Could you check a few things on this model? Use its own coordinates, in mm. Face numbers are marked on the shaded views. A direction names the side the tool comes from. Coordinates: 2 decimals unless noted, no trailing zeros. Order: outer loops, then holes, each group sorted by start corner. A loop starts at its lowest first (then second) coordinate and runs counter-clockwise, first axis right, second up. Notation, with made-up numbers: (-18.75, 80) - (-7.75, 80) arc R30 cw to (-7.75, 113) - close; hole circle Ø10 at (50.5, -30.5). An arc over 180 degrees is marked (long way). Answer as a JSON object with one key per item and string values. Group by question number.
(1) Imagine slicing it at C-C, the plane y = 118. Write out the boundary of the cut face in (x, z), and give its area (3 significant figures).
(2) Please list where these lines run through material, in increasing order: probe 1 along Y at (x, z) = (-6.5, 11); probe 2 along X at (y, z) = (48, -6); probe 3 along X at (y, z) = (30.5, 10).
(3) Imagine slicing it at D-D, the plane x = 8. Write out the boundary of the cut face in (y, z), and give its area (3 significant figures).
(4) Which directions (+Z, -Z, +X, -X, +Y, -Y) give clear straight access to the entire face, cutting with the end or side of a thin tool? Please do the marked faces 1 and 2.
(5) Imagine slicing it at A-A, the plane z = 0. Write out the boundary of the cut face in (x, y), and give its area (3 significant figures).
(6) Will these pins go through, and if not, where does the flat tip stop? P1, Ø17.5, axis at y = 44.5, z = 1, coming from the -X side; P2, Ø6, axis at x = 11, y = 96.5, coming from the +Z side; P3, Ø11, axis at y = 41, z = 1.5, coming from the +X side.
(7) Imagine slicing it at B-B, the plane x = 1.5. Write out the boundary of the cut face in (y, z), and give its area (3 significant figures).
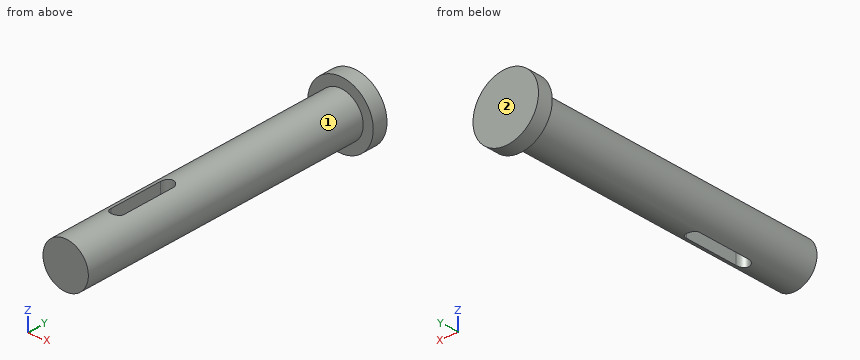
from build123d import *

# Parameters (mm, degrees)
SKETCH1_R           = 11.43
BOSS_EXTRUDE1_DEPTH = 160.02
CUT_EXTRUDE1_DEPTH  = 73.66
BOSS_EXTRUDE2_START = -7.62
SKETCH3_R           = 16.51
SKETCH3_R_2         = 11.43
BOSS_EXTRUDE2_DEPTH = 7.62


with BuildPart() as part:
    # Sketch1 → Boss-Extrude1 (new body)
    with BuildSketch(Plane(origin=(0, 0, 0), x_dir=(1, 0, 0), z_dir=(0, 1, 0))):
        with Locations(Location((0, 0, 0), (0, 0, 270))):
            Circle(SKETCH1_R)
    extrude(amount=BOSS_EXTRUDE1_DEPTH)

    # Sketch2 → Cut-Extrude1 (cut)
    with BuildSketch(Plane.XY.offset(11.43)):
        with BuildLine():
            Line((3.301999683, 28.702000653), (3.301999683, 56.13399967))
            ThreePointArc((3.301999683, 56.13399967), (0, 59.436), (-3.302000317, 56.134000304))
            Line((-3.302000317, 56.134000304), (-3.302000317, 28.702000019))
            ThreePointArc((-3.302000317, 28.702000019), (0, 25.4), (3.301999683, 28.702000653))
        make_face()
    extrude(amount=-CUT_EXTRUDE1_DEPTH, mode=Mode.SUBTRACT)

    # Sketch3 → Boss-Extrude2 (add)
    with BuildSketch(Plane(origin=(0, 160.02, 0), x_dir=(1, 0, 0), z_dir=(0, 1, 0)).offset(BOSS_EXTRUDE2_START)):
        with Locations(Location((0, 0, 0), (0, 0, 270))):
            Circle(SKETCH3_R)
        with Locations(Location((0, 0, 0), (0, 0, 270))):
            Circle(SKETCH3_R_2, mode=Mode.SUBTRACT)
    extrude(amount=BOSS_EXTRUDE2_DEPTH)


solid = part.part
Result set:
{
 "1": {"outline": "circle Ø22.86 at (0, 0)", "area": "410 mm^2"},
 "2": {"probe 1": "y = 152.4 to 160.02", "probe 2": "x = -9.73 to -3.3, 3.3 to 9.73", "probe 3": "x = -5.54 to -3.3, 3.3 to 5.54"},
 "3": {"outline": "(0, -8.16) - (152.4, -8.16) - (152.4, -14.44) - (160.02, -14.44) - (160.02, 14.44) - (152.4, 14.44) - (152.4, 8.16) - (0, 8.16) - close", "area": "2,710 mm^2"},
 "4": {"face 1": "-Y", "face 2": "+Z, -Z, +X, -X, +Y"},
 "5": {"outline": "(-16.51, 152.4) - (-11.43, 152.4) - (-11.43, 0) - (11.43, 0) - (11.43, 152.4) - (16.51, 152.4) - (16.51, 160.02) - (-16.51, 160.02) - close; hole (-3.3, 28.7) arc R3.3 ccw to (3.3, 28.7) - (3.3, 56.13) arc R3.3 ccw to (-3.3, 56.13) - close", "area": "3,520 mm^2"},
 "6": {"P1": "stops at x = -11.43", "P2": "stops at z = 8.16", "P3": "stops at x = 11.43"},
 "7": {"outline": "(0, -11.33) - (25.76, -11.33) - (25.76, 11.33) - (0, 11.33) - close; (59.08, -11.33) - (152.4, -11.33) - (152.4, -16.44) - (160.02, -16.44) - (160.02, 16.44) - (152.4, 16.44) - (152.4, 11.33) - (59.08, 11.33) - close", "area": "2,950 mm^2"}
}
